Verification items for the finished model (mm, model axes). Face numbers are marked on the shaded views. A direction names the side the tool comes from. Round coordinates to 2 decimals unless told otherwise and drop trailing zeros. Order: outer loops, then holes, each group sorted by start corner. A loop starts at its lowest first (then second) coordinate and runs counter-clockwise, first axis right, second up. Notation, with made-up numbers: M 80.5,18 L 94.5,18 A24 ccw 94.5,49 Z; hole C 39.5,53.25 d5. An arc over 180 degrees is marked long. Return JSON: item names as keys, results as strings. Group by question number.
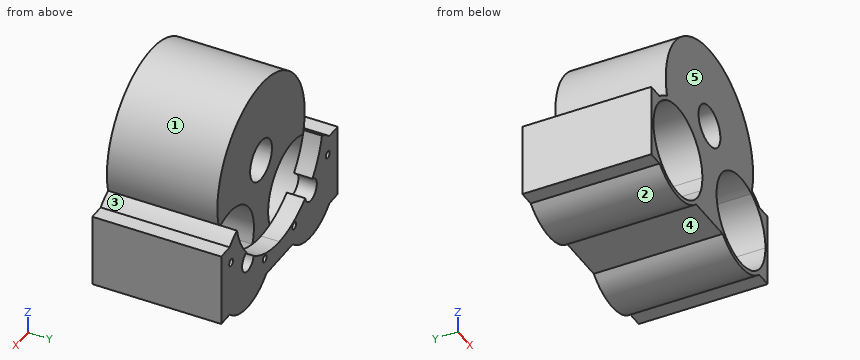
from build123d import *

# Parameters (mm, degrees)
F0_R     = 2.54
F1_DEPTH = 12.7
F2_R     = 14.2875
F3_DEPTH = 76.2


with BuildPart() as f1:
    # F0 (on Front) → F1 (new body)
    with BuildSketch(Plane.XZ):
        with BuildLine():
            Line((0, 50.8), (0, 0))
            Line((0, 0), (10.954276, 0))
            ThreePointArc((10.954276, 0), (34.925, -9.525), (58.895724, 0))
            Line((58.895724, 0), (76.2, 0))
            Line((76.2, 0), (76.2, 13.110851))
            ThreePointArc((76.2, 13.110851), (58.441553, 15.939952), (42.441301, 24.147157))
            ThreePointArc((42.441301, 24.147157), (29.765625, 19.792394), (33.051765, 32.786162))
            ThreePointArc((33.051765, 32.786162), (25.31364, 44.247376), (20.555013, 57.231731))
            ThreePointArc((20.555013, 57.231731), (15.486782, 54.415708), (10.954276, 50.8))
            Line((10.954276, 50.8), (0, 50.8))
        make_face()
        with Locations((56.922045, 12.7)):
            Circle(F0_R, mode=Mode.SUBTRACT)
        with Locations((12.927955, 38.1)):
            Circle(F0_R, mode=Mode.SUBTRACT)
        with BuildLine():
            Line((76.2, 13.110851), (76.2, 0))
            Line((76.2, 0), (93.504276, 0))
            ThreePointArc((93.504276, 0), (117.475, -9.525), (141.445724, 0))
            Line((141.445724, 0), (152.4, 0))
            Line((152.4, 0), (152.4, 50.8))
            Line((152.4, 50.8), (141.445724, 50.8))
            ThreePointArc((141.445724, 50.8), (136.913218, 54.415708), (131.844987, 57.231731))
            ThreePointArc((131.844987, 57.231731), (127.08636, 44.247376), (119.348235, 32.786162))
            ThreePointArc((119.348235, 32.786162), (122.634375, 19.792394), (109.958699, 24.147157))
            ThreePointArc((109.958699, 24.147157), (93.958447, 15.939952), (76.2, 13.110851))
        make_face()
        with Locations((95.477955, 12.7)):
            Circle(F0_R, mode=Mode.SUBTRACT)
        with Locations((139.472045, 38.1)):
            Circle(F0_R, mode=Mode.SUBTRACT)
    extrude(amount=-F1_DEPTH)

    # F2 (on face) → F3 (join)
    with BuildSketch(Plane.XZ):
        with BuildLine():
            ThreePointArc((66.929, 25.4), (66.422356, 19.727915), (64.918467, 14.235415))
            ThreePointArc((64.918467, 14.235415), (70.531278, 13.392687), (76.2, 13.110851))
            ThreePointArc((76.2, 13.110851), (81.868722, 13.392687), (87.481533, 14.235415))
            ThreePointArc((87.481533, 14.235415), (95.805625, 48.951947), (131.0939, 54.361726))
            ThreePointArc((131.0939, 54.361726), (131.488069, 55.791854), (131.844987, 57.231731))
            ThreePointArc((131.844987, 57.231731), (76.2, 127.410851), (20.555013, 57.231731))
            ThreePointArc((20.555013, 57.231731), (20.911931, 55.791854), (21.3061, 54.361726))
            ThreePointArc((21.3061, 54.361726), (52.077212, 52.419579), (66.929, 25.4))
        make_face()
        with Locations((76.2, 70.260851)):
            Circle(F2_R, mode=Mode.SUBTRACT)
        with BuildLine():
            ThreePointArc((76.2, 13.110851), (70.531278, 13.392687), (64.918467, 14.235415))
            ThreePointArc((64.918467, 14.235415), (13.255625, 1.848053), (21.3061, 54.361726))
            ThreePointArc((21.3061, 54.361726), (20.911931, 55.791854), (20.555013, 57.231731))
            ThreePointArc((20.555013, 57.231731), (15.486782, 54.415708), (10.954276, 50.8))
            Line((10.954276, 50.8), (0, 50.8))
            Line((0, 50.8), (0, 0))
            Line((0, 0), (10.954276, 0))
            ThreePointArc((10.954276, 0), (34.925, -9.525), (58.895724, 0))
            Line((58.895724, 0), (76.2, 0))
            Line((76.2, 0), (93.504276, 0))
            ThreePointArc((93.504276, 0), (117.475, -9.525), (141.445724, 0))
            Line((141.445724, 0), (152.4, 0))
            Line((152.4, 0), (152.4, 50.8))
            Line((152.4, 50.8), (141.445724, 50.8))
            ThreePointArc((141.445724, 50.8), (136.913218, 54.415708), (131.844987, 57.231731))
            ThreePointArc((131.844987, 57.231731), (131.488069, 55.791854), (131.0939, 54.361726))
            ThreePointArc((131.0939, 54.361726), (144.494579, 42.552212), (149.479, 25.4))
            ThreePointArc((149.479, 25.4), (123.147085, -6.097356), (87.481533, 14.235415))
            ThreePointArc((87.481533, 14.235415), (81.868722, 13.392687), (76.2, 13.110851))
        make_face()
    extrude(amount=F3_DEPTH)


solid = f1.part
1. Draft check along X on the marked faces 1, 2 and 3. Enter one of: +X half, -X half, draft (parallel to the pull), parting line (faces both ways), or undercut.
2. Thickness scan on line 1 along X through (y, z) = (-49.5, 11.5); line 2 along X through (y, z) = (10, 12); line 3 along X through (y, z) = (3.5, 25.4) (3 decimals). Record the ranges inside material, lowest first. Write a range as from..to.
3. Go/stop test with flat-tipped pins: pin 1 (6 mm diameter, centred on x = 70, y = -37, fed in from -Z); pin 2 (10 mm diameter, centred on y = -24.5, z = 58.5, fed in from -X); pin 3 (6 mm diameter, centred on x = 34, y = -21.5, fed in from +Z). Record where each tip stops, or that it passes through.
4. Cross-section at A-A (y = 5). Enter the section's corners in (x, z) (3 decimals).
5. Cross-section at D-D (y = -34.5). Give the number of separate pieces and of enclosed holes in the cut face, plus the area to 3 significant figures.
6. Cross-section at C-C (z = 38.1). Enter the section's corners in (x, y).
7. Cross-section at B-B (x = 73). Enter the section's corners in (y, z).
8. Access from +Z, -Z, +X, -X, +Y, -Y to the whole of each face (thin tool, end or side, straight path). Record for the marked faces 4 and 5.
Computed:
{
 "1": {"face 1": "parting line", "face 2": "undercut", "face 3": "+X half"},
 "2": {"line 1": "x = 0..6.1, 63.75..88.65, 146.3..152.4", "line 2": "x = 0..54.48, 59.36..93.04, 97.92..152.4", "line 3": "x = 0..27.305, 125.095..152.4"},
 "3": {"pin 1": "stops at z = 0", "pin 2": "stops at x = 14.19", "pin 3": "stops at z = 111.85"},
 "4": {"outline": "M 0,0 L 10.954,0 A34.925 ccw 58.896,0 L 93.504,0 A34.925 ccw 141.446,0 L 152.4,0 L 152.4,50.8 L 141.446,50.8 A34.925 ccw 131.845,57.232 A57.15 cw 119.348,32.786 A7.62 cw long 109.959,24.147 A57.15 cw 42.441,24.147 A7.62 cw long 33.052,32.786 A57.15 cw 20.555,57.232 A34.925 ccw 10.954,50.8 L 0,50.8 Z; hole C 12.928,38.1 d5.08; hole C 56.922,12.7 d5.08; hole C 95.478,12.7 d5.08; hole C 139.472,38.1 d5.08"},
 "5": {"separate pieces": "1", "enclosed holes": "3", "area": "8,680 mm²"},
 "6": {"outline": "M 0,-76.2 L 5.55,-76.2 L 5.55,0 L 10.39,0 L 10.39,12.7 L 0,12.7 Z; M 15.47,0 L 28.96,0 L 28.96,12.7 L 15.47,12.7 Z; M 64.3,-76.2 L 88.1,-76.2 L 88.1,0 L 64.3,0 Z; M 123.44,0 L 136.93,0 L 136.93,12.7 L 123.44,12.7 Z; M 142.01,0 L 146.85,0 L 146.85,-76.2 L 152.4,-76.2 L 152.4,12.7 L 142.01,12.7 Z"},
 "7": {"outline": "M -76.2,0 L 12.7,0 L 12.7,13.2 L 0,13.2 L 0,56.34 L -76.2,56.34 Z; M -76.2,84.19 L 0,84.19 L 0,127.32 L -76.2,127.32 Z"},
 "8": {"face 4": "-Z, +Y, -Y", "face 5": "+Z, -Z, +X, -X, -Y"}
}
